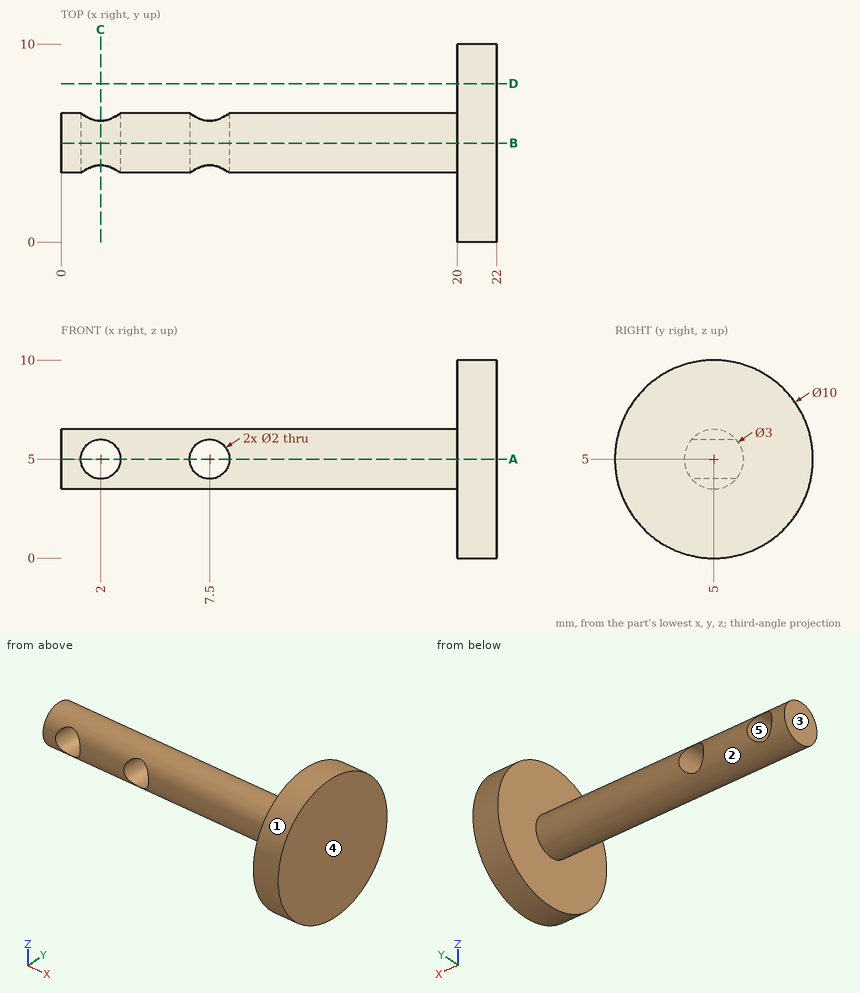
Source: three-view drawing plus pictorial views. Frame: mm from the lowest corner of the part. A direction names the side the tool comes from. Round coordinates to 2 decimals unless told otherwise and drop trailing zeros. Write each loop counter-clockwise with the first axis right and the second up, starting at its lowest first coordinate (ties: lowest second). Pieces come first, ordered by that corner, then holes. Notation, with made-up numbers: M 30.5,-1 L 75.5,-1 A12 cw 75.5,9 Z; hole C 10.5,-32.5 d7. An arc over 180 degrees is marked long. One line per item, written item: value. Start each with the question number.
Item 1: Section query B-B (y = 5). Return the cut outline in (x, z).
Item 2: Section query A-A (z = 5). Return the cut outline in (x, y).
Item 3: Ray query, L1, parallel to X at y = 5.5, z = 5; L2, parallel to X at y = 6, z = 5.5; L3, parallel to X at y = 4, z = 8.75. Return the intervals inside material, ascending. Write a range as from..to.
Item 4: Section query C-C (x = 2). Return the cut outline in (y, z), plus the area to 3 significant figures.
Item 5: Section query D-D (y = 8). Return the cut outline in (x, z), plus the area to 3 significant figures.
Item 6: Pin query (flat end, axial travel): pin 1 (4 mm diameter, centred on x = 14, y = 7, fed in from -Z); pin 2 (4 mm diameter, centred on x = 3, z = 4.5, fed in from -Y); pin 3 (4 mm diameter, centred on x = 15, z = 7.5, fed in from +Y); pin 4 (3 mm diameter, centred on y = 6.5, z = 6, fed in from -X). Return the tip coordinate at first contact, or that it passes through.
Item 7: Set-up query: the marked faces 1 and 2. Return all of +Z, -Z, +X, -X, +Y, -Y with unobstructed straight access to the full face (end or side cutting, diameter ignored); none if empty.
Item 8: Mould query, pull axis X, two halves, no side actions, for the marked faces 3, 4 and 5. Classes: pulls with the +X half, pulls with the -X half, needs draft (parallel to the pull), parting line crosses it, or undercut.
Result set:
1. outline: M 0,3.5 L 20,3.5 L 20,0 L 22,0 L 22,10 L 20,10 L 20,6.5 L 0,6.5 Z; hole C 2,5 d2; hole C 7.5,5 d2
2. outline: M 0,3.5 L 1,3.5 L 1,6.5 L 0,6.5 Z; M 3,3.5 L 6.5,3.5 L 6.5,6.5 L 3,6.5 Z; M 8.5,3.5 L 20,3.5 L 20,0 L 22,0 L 22,10 L 20,10 L 20,6.5 L 8.5,6.5 Z
3. L1: x = 0..1, 3..6.5, 8.5..22
3. L2: x = 0..1.13, 2.87..6.63, 8.37..22
3. L3: x = 20..22
4. outline: M 3.88,4 A1.5 ccw 6.12,4 Z; M 3.88,6 L 6.12,6 A1.5 ccw Z
4. area: 1.55 mm²
5. outline: M 20,1 L 22,1 L 22,9 L 20,9 Z
5. area: 16.0 mm²
6. pin 1: stops at z = 3.5
6. pin 2: stops at y = 3.5
6. pin 3: stops at y = 6.41
6. pin 4: stops at x = 0
7. face 1: +X, -X
7. face 2: -X
8. face 3: pulls with the -X half
8. face 4: pulls with the +X half
8. face 5: undercut
